Input: part model. Units: mm. Frame: model coordinates. Round coordinates to 2 decimals unless told otherwise and drop trailing zeros. Loops run counter-clockwise (first coordinate to the right, second up) from the corner with the lowest first, then second, coordinate; pieces in that order, holes last. Notation, with made-up numbers: M -27,79 L 10,79 A25 cw 10,99 Z; hole C 74,11 d5. An arc over 180 degrees is marked long. Return JSON: item names as keys, results as strings. Group by question number.
1) Section A-A (y = 7). Output: boundary loops of the cut face in (x, z).
2) Section C-C (x = 27). Output: boundary loops of the cut face in (y, z), plus the area to 3 significant figures.
3) Section B-B (z = 2.5). Output: boundary loops of the cut face in (x, y).
4) Material intervals for line 1 (X direction, y = 7, z = 1.9); line 2 (X direction, y = 8, z = 1.8); line 3 (Y direction, x = 5, z = 1.75), sorted ascending. Write a range as from..to.
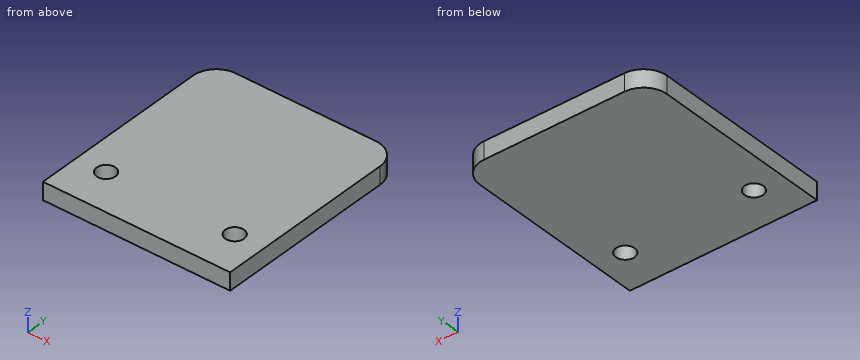
Autodesk Inventor part; units mm, degrees
ref_plane "YZ Plane" through (0, 0, 0) normal (1, 0, 0) x (0, 1, 0)
ref_plane "XZ Plane" through (0, 0, 0) normal (0, 1, 0) x (-1, 0, 0)
ref_plane "XY Plane" through (0, 0, 0) normal (0, 0, 1) x (1, 0, 0)
sketch "Sketch1" plane through (0, 0, 0) normal (0, 0, 1) x (1, 0, 0)
  line L0 (0, 0) -> (32, 0)
  line L1 (32, 0) -> (32, 35)
  line L2 (32, 35) -> (0, 35)
  line L3 (0, 35) -> (0, 0)
  dimension "d0" = 32
  dimension "d1" = 35
extrude "Extrusion1" add sketch "Sketch1" along normal blind 3
sketch "Sketch2" plane through (0, 0, 3) normal (0, 0, 1) x (1, 0, 0)
  line L0 (0, 0) -> (0, 35)
  line L1 (32, 0) -> (0, 0)
  point P0 (5, 7)
  point P1 (27, 7)
  dimension "d4" = 7
  dimension "d5" = 7
  dimension "d6" = 22
  dimension "d7" = 5
hole "Hole1" at (5, 7, 3) at (27, 7, 3) direction (0, 0, -1) diameter 3.2 depth 8 tip angle 118
fillet "Fillet1" radius 4 2 edges at (32, 35, 1.5) (0, 35, 1.5)
properties part number "PLACA" material "Carbon Steel"
Returned:
{
 "1": {"outline": "M 0,0 L 3.4,0 L 3.4,3 L 0,3 Z; M 6.6,0 L 25.4,0 L 25.4,3 L 6.6,3 Z; M 28.6,0 L 32,0 L 32,3 L 28.6,3 Z"},
 "2": {"outline": "M 0,0 L 5.4,0 L 5.4,3 L 0,3 Z; M 8.6,0 L 35,0 L 35,3 L 8.6,3 Z", "area": "95.4 mm^2"},
 "3": {"outline": "M 0,0 L 32,0 L 32,31 A4 ccw 28,35 L 4,35 A4 ccw 0,31 Z; hole C 5,7 d3.2; hole C 27,7 d3.2"},
 "4": {"line 1": "x = 0..3.4, 6.6..25.4, 28.6..32", "line 2": "x = 0..3.75, 6.25..25.75, 28.25..32", "line 3": "y = 0..5.4, 8.6..35"}
}
